Could you check a few things on this drawing? It's one solid part, dimensions in mm from its lowest x, y, z. A direction names the side the tool comes from. Give positions to 0.01 mm unless a question says otherwise; leave off trailing zeros. Write each loop counter-clockwise with the first axis right and the second up, starting at its lowest first coordinate (ties: lowest second). Pieces come first, ordered by that corner, then holes. Notation, with made-up numbers: (-33, 34.25) -> (-5, 34.25) arc R20 cw to (-5, 56.25) -> close; hole circle Ø8 at (54.25, -6). An arc over 180 degrees is marked (long way). Use CSV: the item, a comma, the result in double quotes. Start each with the question number.
(1) Suppose I cut it at C-C on x = 13. List the corners of the cut face in (y, z) for me, plus the area to 3 significant figures.
(2) Which directions (+Z, -Z, +X, -X, +Y, -Y) give clear straight access to the entire face, cutting with the end or side of a thin tool? Please do the marked faces 4 and 5.
(3) Suppose I cut it at D-D on x = 4. List the corners of the cut face in (y, z) for me.
(4) Suppose I cut it at A-A on y = 40. List the corners of the cut face in (x, z) for me.
(5) If we mould it in two halves opening along Z, with no side actions, what happens to the marked faces 1, 2 and 3? For each: pulls with the +Z half, pulls with the -Z half, needs draft (parallel to the pull), parting line crosses it, or undercut.
(6) I need wall thicknesses on L1, parallel to X at y = 29, z = 4; L2, parallel to X at y = 55, z = 55.5; L3, parallel to Z at x = 37, y = 34. Which ranges of each line are inside material? Lowest first, please. Write a range as [from, to].
(7) For pin 1 Ø4 at (x, z) = (18, 16) entering from +Y; pin 2 Ø8 at (x, z) = (34.5, 63) entering from +Y; pin 3 Ø1 at (x, y) = (21.5, 47.5) entering from +Z; pin 4 Ø5 at (y, z) = (40, 40) entering from +X, each with a flat end and sliding along its axis, tell me the tip position at first contact or that it passes through.
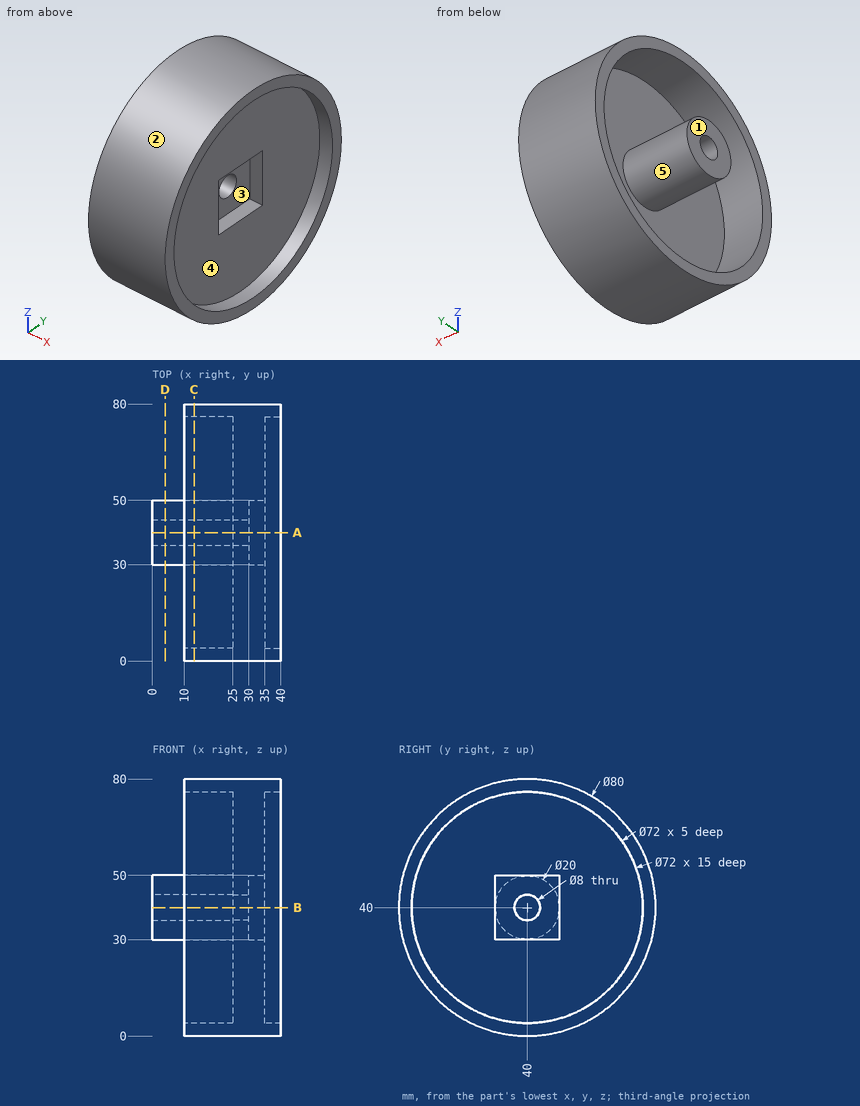
Geometry says:
1,outline,"circle Ø80 at (40, 40); circle Ø20 at (40, 40); hole circle Ø72 at (40, 40); hole circle Ø8 at (40, 40)"
1,area,"1,220 mm²"
2,face 4,"+X"
2,face 5,"-X"
3,outline,"circle Ø20 at (40, 40); hole circle Ø8 at (40, 40)"
4,outline,"(0, 30) -> (25, 30) -> (25, 4) -> (10, 4) -> (10, 0) -> (40, 0) -> (40, 4) -> (35, 4) -> (35, 30) -> (30, 30) -> (30, 36) -> (0, 36) -> close; (0, 44) -> (30, 44) -> (30, 50) -> (35, 50) -> (35, 76) -> (40, 76) -> (40, 80) -> (10, 80) -> (10, 76) -> (25, 76) -> (25, 50) -> (0, 50) -> close"
5,face 1,"needs draft"
5,face 2,"parting line crosses it"
5,face 3,"undercut"
6,L1,"[10, 40]"
6,L2,"[25, 35]"
6,L3,"[0.45, 4.5], [75.5, 79.55]"
7,pin 1,"y = 73.41"
7,pin 2,"y = 75.2"
7,pin 3,"z = 79.38"
7,pin 4,"through"
